```python
from build123d import *

# Parameters (mm, degrees)
ESBO_O1_W                = 41.5
ESBO_O1_H                = 10.2
ESBO_O1_R                = 1.75
RESSALTO_EXTRUS_O1_DEPTH = 2
ESBO_O2_W                = 5.7
ESBO_O2_H                = 10
RESSALTO_EXTRUS_O2_DEPTH = 6
RESSALTO_EXTRUS_O2_TAPER = 10
RESSALTO_EXTRUS_O3_DEPTH = 7.3
CORTE_EXTRUS_O1_START    = -4
CORTE_EXTRUS_O1_DEPTH    = 3.3
RESSALTO_EXTRUS_O4_DEPTH = 3.9
ESBO_O7_W                = 7.5
ESBO_O7_H                = 0.921500294
ESBO_O7_H_2              = 2.228499706
CORTE_EXTRUS_O2_DEPTH    = 2.5
ESBO_O8_R                = 1.75
RESSALTO_EXTRUS_O5_DEPTH = 2.6


with BuildPart() as part:
    # Esboço1 → Ressalto-extrusão1 (new body)
    with BuildSketch(Plane.XY):
        Rectangle(ESBO_O1_W, ESBO_O1_H)
        with Locations((-17.25, 0)):
            Circle(ESBO_O1_R, mode=Mode.SUBTRACT)
        with Locations((-4.45, 0)):
            Circle(ESBO_O1_R, mode=Mode.SUBTRACT)
    extrude(amount=RESSALTO_EXTRUS_O1_DEPTH)

    # Esboço2 → Ressalto-extrusão2 (add)
    with BuildSketch(Plane.XY.offset(2)):
        with Locations((-10.9, 0)):
            Rectangle(ESBO_O2_W, ESBO_O2_H)
    extrude(amount=RESSALTO_EXTRUS_O2_DEPTH, taper=RESSALTO_EXTRUS_O2_TAPER)

    # Esboço3 → Ressalto-extrusão3 (add)
    with BuildSketch(Plane.XY.offset(2)):
        with BuildLine():
            Line((4.25, 3.2), (7.75, 3.2))
            Line((7.75, 3.2), (7.75, -3.2))
            Line((7.75, -3.2), (4.25, -3.2))
            ThreePointArc((4.25, -3.2), (1.05, 0), (4.25, 3.2))
        make_face()
    extrude(amount=RESSALTO_EXTRUS_O3_DEPTH)

    # Esboço4 → Corte-extrusão1 (cut)
    with BuildSketch(Plane.XY.offset(9.3).offset(CORTE_EXTRUS_O1_START)):
        with BuildLine():
            Line((7.05, -3.2), (7.05, -1.7))
            Line((7.05, -1.7), (7.75, -1.7))
            Line((7.75, -1.7), (7.75, 1.7))
            Line((7.75, 1.7), (7.05, 1.7))
            Line((7.05, 1.7), (7.05, 3.2))
            Line((7.05, 3.2), (4.25, 3.2))
            ThreePointArc((4.25, 3.2), (2.270101013, 2.513961018), (1.139131954, 0.75))
            Line((1.139131954, 0.75), (1.839131954, 0.75))
            Line((1.839131954, 0.75), (1.839131954, -0.75))
            Line((1.839131954, -0.75), (1.139131954, -0.75))
            ThreePointArc((1.139131954, -0.75), (2.270101013, -2.513961018), (4.25, -3.2))
            Line((4.25, -3.2), (7.05, -3.2))
        make_face()
    extrude(amount=-CORTE_EXTRUS_O1_DEPTH, mode=Mode.SUBTRACT)

    # Esboço6 → Ressalto-extrusão4 (add, symmetric)
    with BuildSketch(Plane(origin=(0, 0, 0), x_dir=(1, 0, 0), z_dir=(0, 1, 0))):
        Polygon((18.141238668, -2), (18.141238668, -4), (19.195619334, -4), (19.195619334, -6.5), (26.695619334, -6.5), (26.695619334, -6), (19.695619334, -6), (19.695619334, -4), (20.75, -4), (20.75, -2), align=None)
    extrude(amount=RESSALTO_EXTRUS_O4_DEPTH, both=True)

    # Esboço7 → Corte-extrusão2 (cut)
    with BuildSketch(Plane.XY.offset(6.5)):
        with Locations((22.945619334, 3.439249853)):
            Rectangle(ESBO_O7_W, ESBO_O7_H)
        with Locations((22.945619334, 1.364249853)):
            Rectangle(ESBO_O7_W, ESBO_O7_H_2)
        with Locations((22.945619334, -1.364249853)):
            Rectangle(ESBO_O7_W, ESBO_O7_H_2)
        with Locations((22.945619334, -3.439249853)):
            Rectangle(ESBO_O7_W, ESBO_O7_H)
    extrude(amount=-CORTE_EXTRUS_O2_DEPTH, mode=Mode.SUBTRACT)

    # Esboço8 → Ressalto-extrusão5 (add)
    with BuildSketch(Plane(origin=(0, 0, 0), x_dir=(-1, 0, 0), z_dir=(0, 0, -1))):
        Polygon((7.55, 1.789785834), (4.45, 3.579571669), (1.35, 1.789785834), (1.35, -1.789785834), (4.45, -3.579571669), (7.55, -1.789785834), align=None)
        with Locations((4.45, 0)):
            Circle(ESBO_O8_R, mode=Mode.SUBTRACT)
        Polygon((14.15, -1.789785834), (17.25, -3.579571669), (20.35, -1.789785834), (20.35, 1.789785834), (17.25, 3.579571669), (14.15, 1.789785834), align=None)
        with Locations((17.25, 0)):
            Circle(ESBO_O8_R, mode=Mode.SUBTRACT)
    extrude(amount=RESSALTO_EXTRUS_O5_DEPTH)


solid = part.part
```
The model under review builds one solid part; all positions refer to its coordinate system, in mm. A direction names the side the tool comes from. Round coordinates to 2 decimals unless told otherwise and drop trailing zeros. Loops run counter-clockwise (first coordinate to the right, second up) from the corner with the lowest first, then second, coordinate; pieces in that order, holes last. Notation, with made-up numbers: M 15.25,65 L 74.25,65 A18 ccw 74.25,87 Z; hole C -6,53.25 d3. An arc over 180 degrees is marked long. Answer as a JSON object with one key per item and string values.
(1) Tool access review of faces 1 (the flat face through (-18.778, -2.697, -1.282)), 2 (the flat face through (22.1, -2.478, 6.3)), 3 (the flat face through (7.05, 2, 4)): name each direction out of +Z, -Z, +X, -X, +Y, -Y from which nothing blocks a thin tool from reaching the whole face with its end or side.
Resolved:
{"face 1": "-Z, -X, -Y", "face 2": "+Z, +X", "face 3": "+Y, -Y"}
(2) To check wall thickness, follow line 1 along X through (y, z) = (0, -1.9); line 2 along X through (y, z) = (0, 0.95); line 3 along Y through (x, z) = (-4.45, 1.25). State the ranges of each line that lie inside material, in increasing order.
Resolved:
{"line 1": "-20.35 to -19, -15.5 to -14.15, -7.55 to -6.2, -2.7 to -1.35", "line 2": "-20.75 to -19, -15.5 to -6.2, -2.7 to 20.75", "line 3": "-5.1 to -1.75, 1.75 to 5.1"}
(3) Take a section at A-A on x = 22. Give the boundary of the cut face in (y, z), and give its area (3 significant figures).
Resolved:
{"outline": "M -2.98,6 L -2.48,6 L -2.48,6.5 L -2.98,6.5 Z; M -0.25,6 L 0.25,6 L 0.25,6.5 L -0.25,6.5 Z; M 2.48,6 L 2.98,6 L 2.98,6.5 L 2.48,6.5 Z", "area": "0.750 mm²"}
(4) Clearance check with flat-ended pins moving along their axes: P1, Ø2, axis at x = -1, y = 1, coming from the +Z side; P2, Ø5, axis at x = 6.5, y = 2, coming from the -Z side; P3, Ø0.6, axis at y = -0.5, z = 3, coming from the -X side. State where each tip first meets the part, or that it passes through.
Resolved:
{"P1": "z = 2", "P2": "z = 0", "P3": "x = -13.63"}
(5) Take a section at D-D on z = 0.5. Give the boundary of the cut face in (x, y), and give its area (3 significant figures).
Resolved:
{"outline": "M -20.75,-5.1 L 20.75,-5.1 L 20.75,5.1 L -20.75,5.1 Z; hole C -17.25,0 d3.5; hole C -4.45,0 d3.5", "area": "404 mm²"}
(6) Take a section at C-C on z = 2.75. Give the boundary of the cut face in (x, y).
Resolved:
{"outline": "M -13.62,-4.87 L -8.18,-4.87 L -8.18,4.87 L -13.62,4.87 Z; M 1.14,-0.75 L 1.84,-0.75 L 1.84,0.75 L 1.14,0.75 A3.2 ccw Z; M 7.05,-3.2 L 7.75,-3.2 L 7.75,-1.7 L 7.05,-1.7 Z; M 7.05,1.7 L 7.75,1.7 L 7.75,3.2 L 7.05,3.2 Z; M 18.14,-3.9 L 20.75,-3.9 L 20.75,3.9 L 18.14,3.9 Z"}
(7) Draft analysis for pull direction Z (two halves, no side actions). For faces 4 (the flat face through (-18.822, 2.672, -1.282)), 5 (the flat face through (7.05, -2, 4)), 6 (the flat face through (-13.23, -0.07, 4.96)), state which applies: released by +Z, released by -Z, zero draft, split by the parting line, or undercut.
Resolved:
{"face 4": "zero draft", "face 5": "undercut", "face 6": "released by +Z"}
(8) Take a section at B-B on x = 6. Give the boundary of the cut face in (y, z).
Resolved:
{"outline": "M -5.1,0 L 5.1,0 L 5.1,2 L -5.1,2 Z; M -3.2,5.3 L 3.2,5.3 L 3.2,9.3 L -3.2,9.3 Z"}
